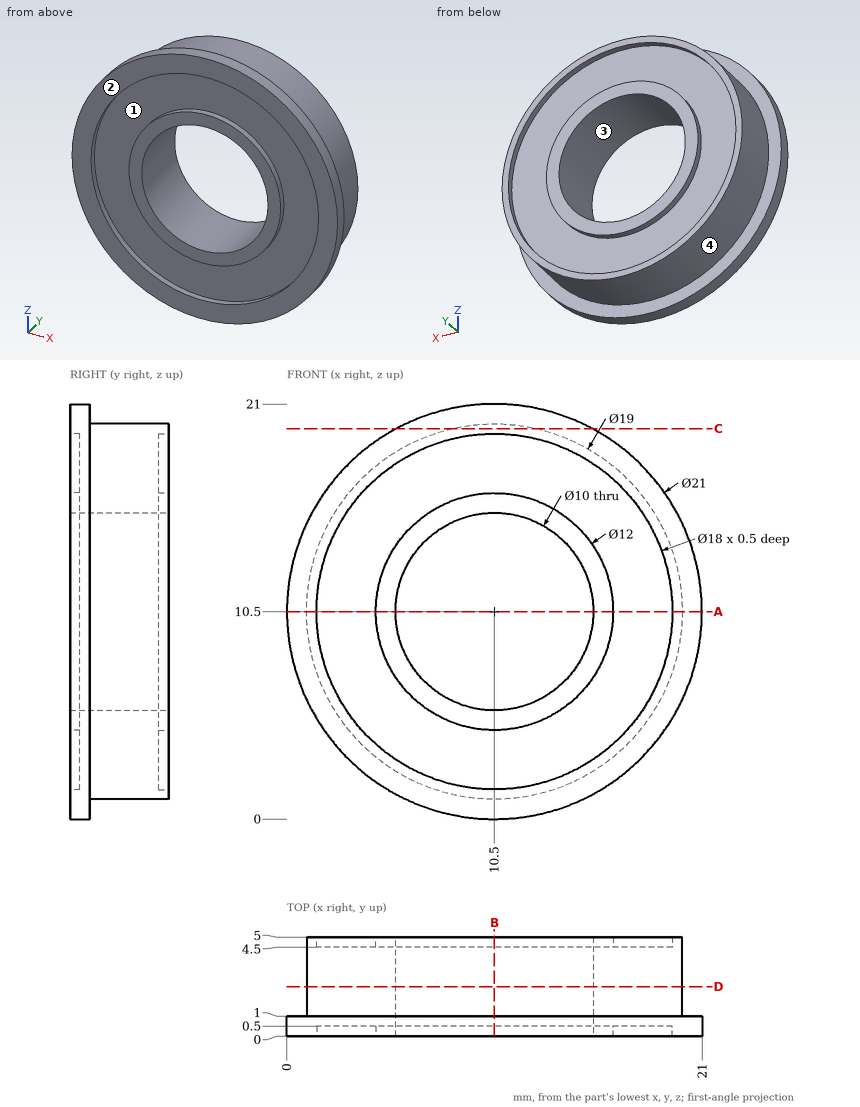
Here's the drawing with two shaded views (mm, measured from the low corner). I have some questions. Coordinates: 2 decimals unless noted, no trailing zeros. Loops run counter-clockwise (first coordinate to the right, second up) from the corner with the lowest first, then second, coordinate; pieces in that order, holes last. Notation, with made-up numbers: (-23, -6.5) -> (-7, -6.5) arc R26 cw to (-7, 10.5) -> close; hole circle Ø7 at (43.25, 83). An arc over 180 degrees is marked (long way). Answer as a JSON object with one key per item and string values.
1) For P1, Ø1, axis at x = 11, z = 4.5, coming from the +Y side; P2, Ø1, axis at x = 17.5, y = 2, coming from the +Z side, each with a flat end and sliding along its axis, tell me the tip position at first contact or that it passes through.
Results:
{"P1": "stops at y = 5", "P2": "stops at z = 17.43"}
2) Imagine slicing it at D-D (y = 2.5). Please give me the cut outline in (x, z), then the cut area to 3 significant figures.
Results:
{"outline": "circle Ø19 at (10.5, 10.5); hole circle Ø10 at (10.5, 10.5)", "area": "205 mm^2"}
3) Imagine slicing it at A-A (z = 10.5). Please give me the cut outline in (x, y).
Results:
{"outline": "(0, 0) -> (1.5, 0) -> (1.5, 0.5) -> (4.5, 0.5) -> (4.5, 0) -> (5.5, 0) -> (5.5, 5) -> (4.5, 5) -> (4.5, 4.5) -> (1.5, 4.5) -> (1.5, 5) -> (1, 5) -> (1, 1) -> (0, 1) -> close; (15.5, 0) -> (16.5, 0) -> (16.5, 0.5) -> (19.5, 0.5) -> (19.5, 0) -> (21, 0) -> (21, 1) -> (20, 1) -> (20, 5) -> (19.5, 5) -> (19.5, 4.5) -> (16.5, 4.5) -> (16.5, 5) -> (15.5, 5) -> close"}
4) Imagine slicing it at C-C (z = 19.75). Please give me the cut outline in (x, y), then the cut area to 3 significant figures.
Results:
{"outline": "(5.53, 0) -> (15.47, 0) -> (15.47, 1) -> (12.67, 1) -> (12.67, 5) -> (8.33, 5) -> (8.33, 1) -> (5.53, 1) -> close", "area": "27.3 mm^2"}
5) Thinking about a two-plate mould opening in X: for the marked faces 1, 2, 3 and 4, which applies, pulls with the +X half, pulls with the -X half, needs draft (parallel to the pull), parting line crosses it, or undercut?
Results:
{"face 1": "undercut", "face 2": "needs draft", "face 3": "undercut", "face 4": "parting line crosses it"}
6) Imagine slicing it at B-B (x = 10.5). Please give me the cut outline in (y, z), then the cut area to 3 significant figures.
Results:
{"outline": "(0, 0) -> (1, 0) -> (1, 1) -> (5, 1) -> (5, 1.5) -> (4.5, 1.5) -> (4.5, 4.5) -> (5, 4.5) -> (5, 5.5) -> (0, 5.5) -> (0, 4.5) -> (0.5, 4.5) -> (0.5, 1.5) -> (0, 1.5) -> close; (0, 15.5) -> (5, 15.5) -> (5, 16.5) -> (4.5, 16.5) -> (4.5, 19.5) -> (5, 19.5) -> (5, 20) -> (1, 20) -> (1, 21) -> (0, 21) -> (0, 19.5) -> (0.5, 19.5) -> (0.5, 16.5) -> (0, 16.5) -> close", "area": "41.0 mm^2"}
7) If I drill on line 1 (Z direction, x = 10.5, y = 0.1); line 2 (Z direction, x = 10.5, y = 4.7); line 3 (Z direction, x = 10.5, y = 1.6), over which ranges is the centre line in solid material (lowest first)?
Results:
{"line 1": "z = 0 to 1.5, 4.5 to 5.5, 15.5 to 16.5, 19.5 to 21", "line 2": "z = 1 to 1.5, 4.5 to 5.5, 15.5 to 16.5, 19.5 to 20", "line 3": "z = 1 to 5.5, 15.5 to 20"}
